Geometry: see drawing. Coordinates: mm, zero at the bounding-box minimum. Round coordinates to 2 decimals unless told otherwise and drop trailing zeros. Write each loop counter-clockwise with the first axis right and the second up, starting at its lowest first coordinate (ties: lowest second). Pieces come first, ordered by that corner, then holes. Notation, with made-up numbers: M 3.5,50.5 L 48.5,50.5 A31 cw 48.5,81.5 Z; hole C 8,45 d5. An arc over 180 degrees is marked long. Write each question's results on one line, items separated by ' | '. Start each with the question number.
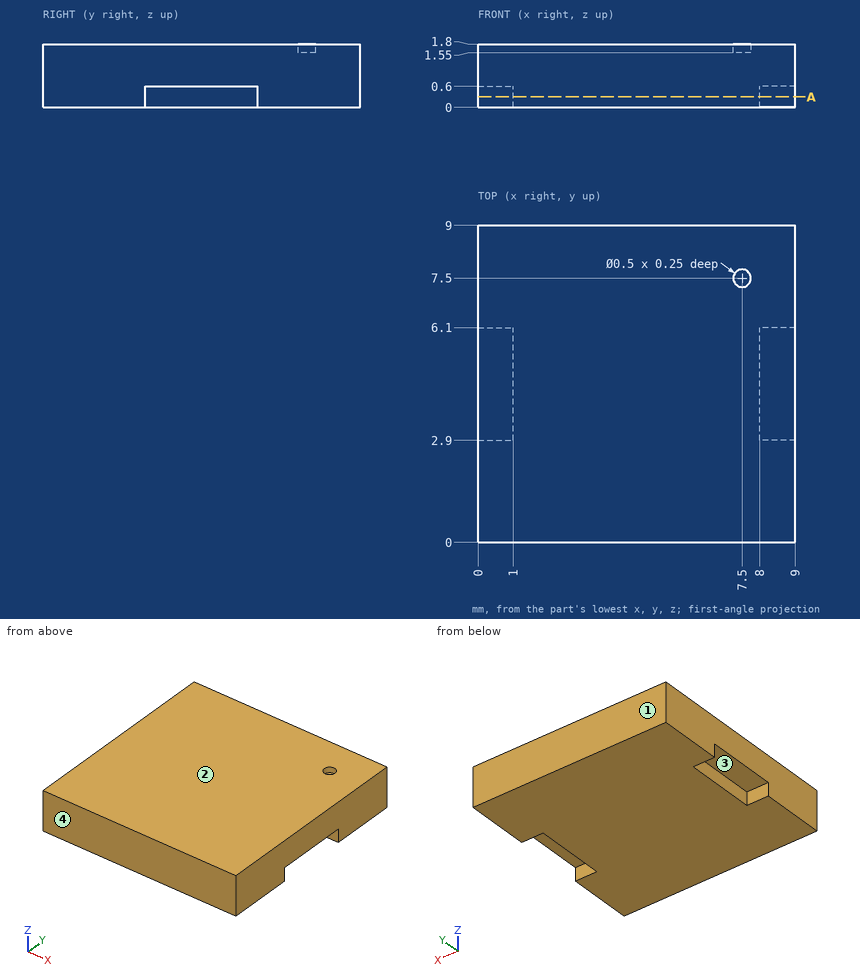
1. Draft query along Y for the marked faces 1, 2, 3 and 4. Return one class per face: +Y half, -Y half, draft (parallel to the pull), parting line (faces both ways), or undercut.
2. Contact query for a flat-ended pin moving along its axis: P1, Ø0.8, axis at x = 0.5, y = 4.5, coming from the -Z side. Output: stop coordinate, or through.
3. Line query: L1, parallel to Y at x = 7.5, z = 1.75; L2, parallel to Y at x = 0.75, z = 0.5; L3, parallel to Z at x = 8.5, y = 5.25. Output: solid intervals per line, ascending. Write a range as from..to.
4. Cut plane A-A on z = 0.3. Output: boundary loops of the cut face in (x, y).
Answers follow:
1) face 1: +Y half | face 2: draft | face 3: undercut | face 4: -Y half
2) P1: stops at z = 0.6
3) L1: y = 0..7.25, 7.75..9 | L2: y = 0..2.9, 6.1..9 | L3: z = 0.6..1.8
4) outline: M 0,0 L 9,0 L 9,2.9 L 8,2.9 L 8,6.1 L 9,6.1 L 9,9 L 0,9 L 0,6.1 L 1,6.1 L 1,2.9 L 0,2.9 Z
